from build123d import *

# Parameters (mm, degrees)
EXTRUDE_1_DEPTH             = 3
HOLE_WIZARD_5_0_5_2_D       = 5
HOLE_WIZARD_3_2_3_2_2_D     = 3.2
PATTERN_LINEAR_1_COUNT      = 3
PATTERN_LINEAR_1_PITCH      = 10
PATTERN_LINEAR_1_COUNT_DIR2 = 2
PATTERN_LINEAR_1_PITCH_DIR2 = 10
SKETCH_8_W                  = 155
SKETCH_8_H                  = 3
EXTRUDE_2_DEPTH             = 13
SKETCH_10_W                 = 50
SKETCH_10_H                 = 3
EXTRUDE_3_DEPTH             = 55
EXTRUDE_5_DEPTH             = 10
SKETCH_12_R                 = 13
CUT_EXTRUDE_1_DEPTH         = 3
SKETCH_13_R                 = 2
CUT_EXTRUDE_2_DEPTH         = 3
PATTERN_CIRCULAR_1_COUNT    = 4
FILLET_1_R                  = 10
HOLE_WIZARD_4_0_4_1_D       = 4


with BuildPart() as part:
    # 草图1 → 凸台-拉伸1 (new body)
    with BuildSketch(Plane(origin=(0, 0, 0), x_dir=(1, 0, 0), z_dir=(0, 1, 0))):
        Polygon((-85, -45), (70, -45), (70, 5), (-70, 45), (-85, 45), align=None)
        Polygon((-85, 45), (-70, 45), (-85, 49.285714286), align=None)
    extrude(amount=EXTRUDE_1_DEPTH)

    # Ø5.0 (5) 直径孔2 (through all)
    with Locations(Plane(origin=(0, 3, 0), x_dir=(1, 0, 0), z_dir=(0, 1, 0))):
        with Locations((-77.5, -37.5), (-77.5, -12.5), (-77.5, 37.5), (-77.5, 12.5)):
            Hole(HOLE_WIZARD_5_0_5_2_D / 2)

    # Ø3.2 (3.2) 直径孔2 (through all)
    with Locations(Plane(origin=(0, 0, 0), x_dir=(-1, 0, 0), z_dir=(0, -1, 0))):
        with Locations((-65, -35)):
            hole_wizard_3_2_3_2_2 = Hole(HOLE_WIZARD_3_2_3_2_2_D / 2)

    # 阵列(线性)1: Hole Wizard 3.2 _3.2_ _2 3 × 2
    with Locations(*[(-j * PATTERN_LINEAR_1_PITCH_DIR2, 0, -i * PATTERN_LINEAR_1_PITCH) for i in range(PATTERN_LINEAR_1_COUNT) for j in range(PATTERN_LINEAR_1_COUNT_DIR2) if (i, j) != (0, 0)]):
        add(hole_wizard_3_2_3_2_2, mode=Mode.SUBTRACT)

    # 草图8 → 凸台-拉伸2 (add)
    with BuildSketch(Plane(origin=(0, 3, 0), x_dir=(1, 0, 0), z_dir=(0, 1, 0))):
        with Locations((-7.5, -46.5)):
            Rectangle(SKETCH_8_W, SKETCH_8_H)
    extrude(amount=-EXTRUDE_2_DEPTH)

    # 草图10 → 凸台-拉伸3 (add)
    with BuildSketch(Plane(origin=(0, 3, 0), x_dir=(1, 0, 0), z_dir=(0, 1, 0))):
        with Locations((5, -46.5)):
            Rectangle(SKETCH_10_W, SKETCH_10_H)
    extrude(amount=-EXTRUDE_3_DEPTH)

    # 草图11 → 凸台-拉伸5 (add)
    with BuildSketch(Plane(origin=(0, 0, 0), x_dir=(1, 0, 0), z_dir=(0, 1, 0))):
        Polygon((-85, 49.285714286), (-84.175836616, 52.170286129), (70.824163384, 7.884571843), (70, 5), align=None)
    extrude(amount=EXTRUDE_5_DEPTH)

    # 草图12 → 切除-拉伸1 (cut)
    with BuildSketch(Plane.XY.offset(48)):
        with Locations((5, -27)):
            Circle(SKETCH_12_R)
    extrude(amount=-CUT_EXTRUDE_1_DEPTH, mode=Mode.SUBTRACT)

    # 草图13 → 切除-拉伸2 (cut)
    with BuildSketch(Plane.XY.offset(48)):
        with Locations((5, -44.5)):
            Circle(SKETCH_13_R)
    cut_extrude_2 = extrude(amount=-CUT_EXTRUDE_2_DEPTH, mode=Mode.SUBTRACT)

    # 阵列(圆周)1: 切除-拉伸2 ×4 about axis
    pattern_circular_1_axis = Axis((5, -27, 0), (0, 0, 1))
    for i in range(1, PATTERN_CIRCULAR_1_COUNT):
        add(cut_extrude_2.rotate(pattern_circular_1_axis, i * 360 / PATTERN_CIRCULAR_1_COUNT), mode=Mode.SUBTRACT)

    # 圆角1
    fillet_1_edges = [part.edges().sort_by_distance(p)[0] for p in [
        (-20, -10, 46.5),
        (30, -10, 46.5),
        (30, -52, 46.5),
        (-20, -52, 46.5),
    ]]
    fillet(fillet_1_edges, radius=FILLET_1_R)

    # Ø4.0 (4) 直径孔1 (through all)
    with Locations(Plane(origin=(0, 0, 0), x_dir=(-1, 0, 0), z_dir=(0, -1, 0))):
        with Locations((16, -1), (-26, -23), (16, -23), (-26, -1)):
            Hole(HOLE_WIZARD_4_0_4_1_D / 2)


solid = part.part
Can you work these out from the model? Positions are in its coordinate system, mm. A direction names the side the tool comes from. Coordinates: 2 decimals unless noted, no trailing zeros. Order: outer loops, then holes, each group sorted by start corner. A loop starts at its lowest first (then second) coordinate and runs counter-clockwise, first axis right, second up. Notation, with made-up numbers: (17, 26.5) -> (30, 26.5) arc R20 cw to (30, 40.5) -> close; hole circle Ø2 at (-35, 7). An arc over 180 degrees is marked (long way). Use one line per item in the form item = value.
Q1. We'd pull the mould along X, two halves only. Please class faces 1 (the face through (56.526, 1.521, 24.519)), 2 (the face through (33.01, -12.85, 46.48)), 3 (the face through (-23.01, -12.85, 46.48)): released by +X, released by -X, zero draft, split by the parting line, or undercut.
From the geometry:
face_1 = undercut
face_2 = released by +X
face_3 = released by -X
Q2. Imagine slicing it at A-A, the plane y = -27. List the corners of the cut face in (x, z) for me, then the cut area to 3 significant figures.
From the geometry:
outline = (-20, 45) -> (-14.5, 45) -> (-14.5, 48) -> (-20, 48) -> close; (-10.5, 45) -> (-8, 45) -> (-8, 48) -> (-10.5, 48) -> close; (18, 45) -> (20.5, 45) -> (20.5, 48) -> (18, 48) -> close; (24.5, 45) -> (30, 45) -> (30, 48) -> (24.5, 48) -> close
area = 48.0 mm²
Q3. Imagine slicing it at C-C, the plane x = -77.5. List the corners of the cut face in (y, z) for me.
From the geometry:
outline = (-10, 45) -> (0, 45) -> (0, 40) -> (3, 40) -> (3, 48) -> (-10, 48) -> close; (0, -50.26) -> (10, -50.26) -> (10, -47.14) -> (3, -47.14) -> (3, -40) -> (0, -40) -> close; (0, -35) -> (3, -35) -> (3, -15) -> (0, -15) -> close; (0, -10) -> (3, -10) -> (3, 10) -> (0, 10) -> close; (0, 15) -> (3, 15) -> (3, 35) -> (0, 35) -> close
Q4. Imagine slicing it at D-D, the plane x = -60. List the corners of the cut face in (y, z) for me, then the cut area to 3 significant figures.
From the geometry:
outline = (-10, 45) -> (0, 45) -> (0, -45.26) -> (10, -45.26) -> (10, -42.14) -> (3, -42.14) -> (3, 48) -> (-10, 48) -> close
area = 332 mm²
Q5. I need wall thicknesses on L1, parallel to Y at x = 5, z = 47.1; L2, parallel to X at y = 1.45, z = 12.5; L3, parallel to Z at x = -77, y = 1. Which ranges of each line are inside material? Lowest first, please.
From the geometry:
L1 = -52 to -46.5, -42.5 to -40, -14 to -11.5, -7.5 to 3
L2 = -85 to -80, -75 to 70
L3 = -50.12 to -39.95, -35.05 to -14.95, -10.05 to 10.05, 14.95 to 35.05, 39.95 to 48
Q6. Imagine slicing it at B-B, the plane y = -36. List the corners of the cut face in (x, z) for me, then the cut area to 3 significant figures.
From the geometry:
outline = (-20, 45) -> (-4.38, 45) -> (-4.38, 48) -> (-20, 48) -> close; (14.38, 45) -> (30, 45) -> (30, 48) -> (14.38, 48) -> close
area = 93.7 mm²
Q7. Which directions (+Z, -Z, +X, -X, +Y, -Y) give clear straight access to the entire face, cutting with the end or side of a thin tool? Please do faces 4 (the face through (-9, 3, 9)), 5 (the face through (-13.266, -28.847, 46.521)), 6 (the face through (-58, -10, 46)).
From the geometry:
face_4 = +Z, -X, +Y
face_5 = +Z, -Z
face_6 = +Z, -Z, -X, -Y
Q8. Will these pins go through, and if not, where does the flat tip stop? P1, Ø2, axis at x = -46, z = 15.5, coming from the +Y side; P2, Ø14.5, axis at y = -2.5, z = 11.5, coming from the +X side; P3, Ø6.5, axis at x = 5, y = -9.5, coming from the -Z side; P4, Ø3, axis at x = 6, y = -15.5, coming from the +Z side.
From the geometry:
P1 = 3
P2 = 70
P3 = 45
P4 = 48
